Source: CAD feature listing. Evaluate the final solid. Frame: model axes, mm. A direction names the side the tool comes from. Round coordinates to 2 decimals unless told otherwise and drop trailing zeros. Write each loop counter-clockwise with the first axis right and the second up, starting at its lowest first coordinate (ties: lowest second). Pieces come first, ordered by that corner, then holes. Notation, with made-up numbers: M -6,47.5 L 36,47.5 A21 ccw 36,58.5 Z; hole C -8,31 d7. An arc over 180 degrees is marked long. Use a Markdown table: item, result.
```python
from build123d import *
from OCP.BRepFilletAPI import BRepFilletAPI_MakeChamfer

# Parameters (mm, degrees)
CROQUIS1_W              = 105
CROQUIS1_H              = 150
SALIENTE_EXTRUIR1_DEPTH = 8
CROQUIS2_R              = 2.9
CORTAR_EXTRUIR4_DEPTH   = 8
CROQUIS3_W              = 58
CROQUIS3_H              = 27
SALIENTE_EXTRUIR2_DEPTH = 6
REDONDEO1_R             = 8
REDONDEO2_R             = 8
REDONDEO3_R             = 8
REDONDEO4_R             = 8
CORTAR_EXTRUIR5_DEPTH   = 2
CHAFL_N1_SIZE           = 2
CHAFL_N1_SIZE2          = 1.154700538
CHAFL_N2_SIZE           = 2
CHAFL_N2_SIZE2          = 3.464101615
CORTAR_EXTRUIR6_DEPTH   = 8


with BuildPart() as part:
    # Croquis1 → Saliente-Extruir1 (new body)
    with BuildSketch(Plane.XY):
        with Locations((52.5, 75)):
            Rectangle(CROQUIS1_W, CROQUIS1_H)
    extrude(amount=SALIENTE_EXTRUIR1_DEPTH)

    # Croquis2 → Cortar-Extruir4 (cut)
    with BuildSketch(Plane.XY.offset(8)):
        with Locations((52.5, 137)):
            Circle(CROQUIS2_R)
        with BuildLine():
            Line((19.25, 108), (19.25, 15))
            ThreePointArc((19.25, 15), (15, 10.75), (10.75, 15))
            Line((10.75, 15), (10.75, 108))
            ThreePointArc((10.75, 108), (15, 112.25), (19.25, 108))
        make_face()
        with BuildLine():
            Line((85.75, 108), (85.75, 15))
            ThreePointArc((85.75, 15), (90, 10.75), (94.25, 15))
            Line((94.25, 15), (94.25, 108))
            ThreePointArc((94.25, 108), (90, 112.25), (85.75, 108))
        make_face()
    extrude(amount=-CORTAR_EXTRUIR4_DEPTH, mode=Mode.SUBTRACT)

    # Croquis3 → Saliente-Extruir2 (add)
    with BuildSketch(Plane.XY.offset(8)):
        with Locations((52.5, 136.5)):
            Rectangle(CROQUIS3_W, CROQUIS3_H)
        Polygon((77.5, 127), (52.5, 127), (27.5, 127), (27.5, 147.5), (77.5, 147.5), align=None, mode=Mode.SUBTRACT)
    extrude(amount=SALIENTE_EXTRUIR2_DEPTH)

    # Redondeo1
    redondeo1_edges = [part.edges().sort_by_distance(p)[0] for p in [
        (0, 150, 4),
    ]]
    fillet(redondeo1_edges, radius=REDONDEO1_R)

    # Redondeo2
    redondeo2_edges = [part.edges().sort_by_distance(p)[0] for p in [
        (105, 150, 4),
    ]]
    fillet(redondeo2_edges, radius=REDONDEO2_R)

    # Redondeo3
    redondeo3_edges = [part.edges().sort_by_distance(p)[0] for p in [
        (0, 0, 4),
    ]]
    fillet(redondeo3_edges, radius=REDONDEO3_R)

    # Redondeo4
    redondeo4_edges = [part.edges().sort_by_distance(p)[0] for p in [
        (105, 0, 4),
    ]]
    fillet(redondeo4_edges, radius=REDONDEO4_R)

    # Croquis4 → Cortar-Extruir5 (cut)
    # profile 1 of 2: a face of its own
    with BuildSketch(Plane.XY.offset(8)):
        with BuildLine():
            Line((27, 108), (27, 15))
            ThreePointArc((27, 15), (15, 3), (3, 15))
            Line((3, 15), (3, 108))
            ThreePointArc((3, 108), (15, 120), (27, 108))
        make_face()
        with BuildLine():
            Line((10.75, 108), (10.75, 15))
            ThreePointArc((10.75, 15), (15, 10.75), (19.25, 15))
            Line((19.25, 15), (19.25, 108))
            ThreePointArc((19.25, 108), (15, 112.25), (10.75, 108))
        make_face(mode=Mode.SUBTRACT)
    # profile 2 of 2: a face of its own
    with BuildSketch(Plane.XY.offset(8)):
        with BuildLine():
            Line((78, 108), (78, 15))
            ThreePointArc((78, 15), (90, 3), (102, 15))
            Line((102, 15), (102, 108))
            ThreePointArc((102, 108), (90, 120), (78, 108))
        make_face()
        with BuildLine():
            Line((85.75, 108), (85.75, 15))
            ThreePointArc((85.75, 15), (90, 10.75), (94.25, 15))
            Line((94.25, 15), (94.25, 108))
            ThreePointArc((94.25, 108), (90, 112.25), (85.75, 108))
        make_face(mode=Mode.SUBTRACT)
    extrude(amount=-CORTAR_EXTRUIR5_DEPTH, mode=Mode.SUBTRACT)

    # Chaflán1: one chamfer whose edges measure the first distance from different faces: ONE call of the kernel's chamfer builder (chamfer() names one face for all edges)
    chafl_n1_edges_1 = [part.edges().sort_by_distance(p)[0] for p in [
        (52.5, 127, 14),
    ]]
    chafl_n1_side_1 = [part.faces().sort_by_distance(p)[0] for p in [
        (52.5, 127, 11),
    ]]
    chafl_n1_edges_2 = [part.edges().sort_by_distance(p)[0] for p in [
        (27.5, 137.25, 14),
    ]]
    chafl_n1_side_2 = [part.faces().sort_by_distance(p)[0] for p in [
        (27.5, 137.25, 11),
    ]]
    chafl_n1_edges_3 = [part.edges().sort_by_distance(p)[0] for p in [
        (52.5, 147.5, 14),
    ]]
    chafl_n1_side_3 = [part.faces().sort_by_distance(p)[0] for p in [
        (52.5, 147.5, 11),
    ]]
    chafl_n1_edges_4 = [part.edges().sort_by_distance(p)[0] for p in [
        (77.5, 137.25, 14),
    ]]
    chafl_n1_side_4 = [part.faces().sort_by_distance(p)[0] for p in [
        (77.5, 137.25, 11),
    ]]
    chafl_n1 = BRepFilletAPI_MakeChamfer(part.part.solid().wrapped)
    for e in chafl_n1_edges_1:
        chafl_n1.Add(CHAFL_N1_SIZE, CHAFL_N1_SIZE2, e.wrapped, chafl_n1_side_1[0].wrapped)  # the first distance lies on this face
    for e in chafl_n1_edges_2:
        chafl_n1.Add(CHAFL_N1_SIZE, CHAFL_N1_SIZE2, e.wrapped, chafl_n1_side_2[0].wrapped)  # the first distance lies on this face
    for e in chafl_n1_edges_3:
        chafl_n1.Add(CHAFL_N1_SIZE, CHAFL_N1_SIZE2, e.wrapped, chafl_n1_side_3[0].wrapped)  # the first distance lies on this face
    for e in chafl_n1_edges_4:
        chafl_n1.Add(CHAFL_N1_SIZE, CHAFL_N1_SIZE2, e.wrapped, chafl_n1_side_4[0].wrapped)  # the first distance lies on this face
    add(Compound.cast(chafl_n1.Shape()), mode=Mode.REPLACE)

    # Chaflán2
    chafl_n2_edges = [part.edges().sort_by_distance(p)[0] for p in [
        (52.5, 123, 8),
        (81.5, 136.5, 8),
        (23.5, 136.5, 8),
    ]]
    chafl_n2_side = [part.faces().sort_by_distance(p)[0] for p in [
        (52.5, 72.279712642, 8),
    ]]
    chamfer(chafl_n2_edges, length=CHAFL_N2_SIZE, length2=CHAFL_N2_SIZE2, reference=chafl_n2_side[0])

    # Croquis6 → Cortar-Extruir6 (cut)
    with BuildSketch(Plane.XY.offset(8)):
        with BuildLine():
            Line((37, 20), (68, 20))
            ThreePointArc((68, 20), (70.5, 17.5), (68, 15))
            Line((68, 15), (37, 15))
            ThreePointArc((37, 15), (34.5, 17.5), (37, 20))
        make_face()
        with BuildLine():
            Line((37, 30), (68, 30))
            ThreePointArc((68, 30), (70.5, 32.5), (68, 35))
            Line((68, 35), (37, 35))
            ThreePointArc((37, 35), (34.5, 32.5), (37, 30))
        make_face()
        with BuildLine():
            Line((37, 45), (68, 45))
            ThreePointArc((68, 45), (70.5, 47.5), (68, 50))
            Line((68, 50), (37, 50))
            ThreePointArc((37, 50), (34.5, 47.5), (37, 45))
        make_face()
        with BuildLine():
            Line((37, 60), (68, 60))
            ThreePointArc((68, 60), (70.5, 62.5), (68, 65))
            Line((68, 65), (37, 65))
            ThreePointArc((37, 65), (34.5, 62.5), (37, 60))
        make_face()
        with BuildLine():
            Line((37, 75), (68, 75))
            ThreePointArc((68, 75), (70.5, 77.5), (68, 80))
            Line((68, 80), (37, 80))
            ThreePointArc((37, 80), (34.5, 77.5), (37, 75))
        make_face()
        with BuildLine():
            Line((37, 90), (68, 90))
            ThreePointArc((68, 90), (70.5, 92.5), (68, 95))
            Line((68, 95), (37, 95))
            ThreePointArc((37, 95), (34.5, 92.5), (37, 90))
        make_face()
        with BuildLine():
            Line((37, 105), (68, 105))
            ThreePointArc((68, 105), (70.5, 107.5), (68, 110))
            Line((68, 110), (37, 110))
            ThreePointArc((37, 110), (34.5, 107.5), (37, 105))
        make_face()
    extrude(amount=-CORTAR_EXTRUIR6_DEPTH, mode=Mode.SUBTRACT)


solid = part.part
```
Q1. Section B-B on y = 77.5. Return loops of the section in (x, z).
Results are:
| item | result |
|---|---|
| outline | M 0,0 L 10.75,0 L 10.75,6 L 3,6 L 3,8 L 0,8 Z; M 19.25,0 L 34.5,0 L 34.5,8 L 27,8 L 27,6 L 19.25,6 Z; M 70.5,0 L 85.75,0 L 85.75,6 L 78,6 L 78,8 L 70.5,8 Z; M 94.25,0 L 105,0 L 105,8 L 102,8 L 102,6 L 94.25,6 Z |
Q2. Section D-D on x = 72. Return loops of the section in (y, z).
Results are:
| item | result |
|---|---|
| outline | M 0,0 L 150,0 L 150,14 L 148.65,14 L 147.5,12 L 147.5,8 L 127,8 L 127,12 L 125.85,14 L 123,14 L 123,11.46 L 121,8 L 0,8 Z |
Q3. Mould query, pull axis Y, two halves, no side actions, for faces 4 (the flat face through (52.4, 125.6, 14)), 5 (the flat face through (52, 0, 4)), 6 (the flat face through (52, 90, 4)), 7 (the flat face through (53, 35, 4)). Classes: +Y half, -Y half, draft (parallel to the pull), parting line (faces both ways), or undercut.
Results are:
| item | result |
|---|---|
| face 4 | draft |
| face 5 | -Y half |
| face 6 | undercut |
| face 7 | undercut |
Q4. Section A-A on x = 15. Return loops of the section in (y, z), plus the area to 3 significant figures.
Results are:
| item | result |
|---|---|
| outline | M 0,0 L 10.75,0 L 10.75,6 L 3,6 L 3,8 L 0,8 Z; M 112.25,0 L 150,0 L 150,8 L 120,8 L 120,6 L 112.25,6 Z |
| area | 357 mm^2 |
Q5. Section C-C on y = 36.5. Return loops of the section in (x, z).
Results are:
| item | result |
|---|---|
| outline | M 0,0 L 10.75,0 L 10.75,6 L 3,6 L 3,8 L 0,8 Z; M 19.25,0 L 85.75,0 L 85.75,6 L 78,6 L 78,8 L 27,8 L 27,6 L 19.25,6 Z; M 94.25,0 L 105,0 L 105,8 L 102,8 L 102,6 L 94.25,6 Z |
Q6. Line query: L1, parallel to X at y = 119, z = 6.5; L2, parallel to X at y = 72, z = 6.5; L3, parallel to X at y = 137, z = 5.75. Output: solid intervals per line, ascending.
Results are:
| item | result |
|---|---|
| L1 | 0 to 10.2, 19.8 to 85.2, 94.8 to 105 |
| L2 | 0 to 3, 27 to 78, 102 to 105 |
| L3 | 0 to 49.6, 55.4 to 105 |
Q7. Reachability of faces 1 (the flat face through (27.5, 137, 10)), 2 (the flat face through (53, 50, 4)), 3 (the flat face through (22.514, 135.297, 9.756)) from +Z, -Z, +X, -X, +Y, -Y: full face, straight path, thin tool, end or side. Return the list, or none.
Results are:
| item | result |
|---|---|
| face 1 | +Z |
| face 2 | +Z, -Z |
| face 3 | +Z, -X, +Y, -Y |
Q8. First-contact query: pin 1 Ø10 at (x, y) = (79.5, 105) entering from +Z; pin 2 Ø1.2 at (x, z) = (49, 9) entering from -Y; pin 3 Ø0.8 at (y, z) = (138, 12) entering from -X. Flat tips, straight axial feed; report the tip coordinate or a pass-through.
Results are:
| item | result |
|---|---|
| pin 1 | z = 8 |
| pin 2 | y = 121.23 |
| pin 3 | x = 23.5 |
